```python
from build123d import *

# Parameters (mm, degrees)
CHAMFER1_SIZE          = 1
MOVE_START             = -5
MOVE_FACE1_OUTLINE_R   = 12.65
MOVE_FACE1_OUTLINE_R_2 = 12.5
MOVE_FACE1_OUTLINE_R_3 = 10.5
MOVE_FACE1_OUTLINE_R_4 = 10.35
MOVE_FACE1_DEPTH       = 22
SKETCH2_W              = 3
SKETCH2_H              = 0.5
LPATTERN1_COUNT        = 15
LPATTERN1_PITCH        = 1.25


with BuildPart() as part:
    # Sketch1 → Revolve1 (revolve)
    with BuildSketch(Plane.XY, mode=Mode.PRIVATE) as revolve1_sk:
        with BuildLine():
            Line((0, -15), (0, 17))
            Line((0, 17), (10.5, 17))
            Line((10.5, 17), (10.5, -5))
            Line((10.5, -5), (12.5, -5))
            Line((12.5, -5), (12.5, 9.5))
            Line((12.5, 9.5), (14.696938457, 9.5))
            ThreePointArc((14.696938457, 9.5), (17.047381221, -3.954338567), (9.013878189, -15))
            Line((9.013878189, -15), (0, -15))
        make_face()
    revolve(revolve1_sk.sketch.rotate(Axis((0, -15, 0), (0, 1, 0)), 90), axis=Axis((0, -15, 0), (0, 1, 0)))

    # Chamfer1
    # the kernel refuses this chamfer: 3.367367181, 1 mm, written as the material it takes off along each edge
    with BuildSketch(Plane(origin=(0, 17, 0), x_dir=(0, 0, -1), z_dir=(1, 0, 0))) as chamfer1_piece_1:
        Polygon((10.5 - CHAMFER1_SIZE, 0), (10.5, -CHAMFER1_SIZE), (10.5, 0), align=None)
    revolve(axis=Axis((0, 17, 0), (0, 1, 0)), mode=Mode.SUBTRACT)
    with BuildSketch(Plane(origin=(0, 9.5, 0), x_dir=(0, 0, -1), z_dir=(1, 0, 0))) as chamfer1_piece_2:
        Polygon((12.5, -CHAMFER1_SIZE), (12.5 + CHAMFER1_SIZE, 0), (12.5, 0), align=None)
    revolve(axis=Axis((0, 9.5, 0), (0, 1, 0)), mode=Mode.SUBTRACT)
    with BuildSketch(Plane(origin=(0, 9.5, 0), x_dir=(0, 0, -1), z_dir=(1, 0, 0))) as chamfer1_piece_3:
        with BuildLine():
            Line((14.696938457 - CHAMFER1_SIZE, 0), (15.911300266, -2.214361809))
            ThreePointArc((15.911300266, -2.214361809), (15.375147387, -1.142079038), (14.696938457, 0))
            Line((14.696938457, 0), (14.696938457 - CHAMFER1_SIZE, 0))
        make_face()
    revolve(axis=Axis((0, 9.5, 0), (0, 1, 0)), mode=Mode.SUBTRACT)

    # Move Face1: read off the stored shape, not the designer's step
    # Move Face1 outline → Move Face1 (cut)
    # profile 1 of 2: a face of its own
    with BuildSketch(Plane(origin=(0, 0, 0), x_dir=(1, 0, 0), z_dir=(0, 1, 0)).offset(MOVE_START)):
        Circle(MOVE_FACE1_OUTLINE_R)
        Circle(MOVE_FACE1_OUTLINE_R_2, mode=Mode.SUBTRACT)
    # profile 2 of 2: a face of its own
    with BuildSketch(Plane(origin=(0, 0, 0), x_dir=(1, 0, 0), z_dir=(0, 1, 0)).offset(MOVE_START)):
        Circle(MOVE_FACE1_OUTLINE_R_3)
        Circle(MOVE_FACE1_OUTLINE_R_4, mode=Mode.SUBTRACT)
    extrude(amount=MOVE_FACE1_DEPTH, mode=Mode.SUBTRACT)

    # Sketch2 → Cut-Revolve1 (revolve, cut)
    with BuildSketch(Plane.XY):
        with Locations((11.5, 14.4)):
            Rectangle(SKETCH2_W, SKETCH2_H)
    cut_revolve1 = revolve(axis=Axis((0, 0, 0), (0, 1, 0)), mode=Mode.SUBTRACT)

    # LPattern1: Cut-Revolve1 ×15
    with Locations(*[(0, -i * LPATTERN1_PITCH, 0) for i in range(1, LPATTERN1_COUNT)]):
        add(cut_revolve1, mode=Mode.SUBTRACT)


solid = part.part
```
Check sheet for the modelled part. Datum: model origin and axes. Units: mm. A direction names the side the tool comes from. Give positions to 0.01 mm unless a question says otherwise; leave off trailing zeros. Order: outer loops, then holes, each group sorted by start corner. A loop starts at its lowest first (then second) coordinate and runs counter-clockwise, first axis right, second up. Notation, with made-up numbers: M 2.25,60 L 21.25,60 A14 ccw 21.25,83 Z; hole C -39,43.5 d11. An arc over 180 degrees is marked long. Answer in a Markdown table with one row per item. Add a question column.
Q1. Gauge pin test, flat ends, axial feed: pin 1 Ø1 at (x, z) = (7.5, -10) entering from -Y; pin 2 Ø1.5 at (y, z) = (1.5, -1) entering from -X; pin 3 Ø2 at (x, z) = (13, 7.5) entering from +Y. Record the tip position at first contact, or that the pin passes through.
Q2. Release check for a two-part mould opening along Y. For faces 1 (the cylindrical face through (-2.74, -1.23, 12.35)), 2 (the conical face through (5, 9, -12)), 3 (the cylindrical face through (-2.17, 10.65, 9.76)) record: released by +Y, released by -Y, zero draft, split by the parting line, or undercut.
Q3. Thickness scan on L1, parallel to Z at x = -8.5, y = 2; L2, parallel to X at y = 1.8, z = 0; L3, parallel to X at y = 0, z = -6. Record the ranges inside material, lowest first.
Q4. Access from +Z, -Z, +X, -X, +Y, -Y to the whole of each face (thin tool, end or side, straight path). Record for faces 4 (the cylindrical face through (-2.17, -1.85, 9.76)), 5 (the cylindrical face through (-2.74, 3.77, 12.35)).
Q5. Sectioned sample at A-A, the plane y = -9.5. Record the boundary of the cut face in (x, z), and give its area (3 significant figures).
Verdict:
| question | item | result |
|---|---|---|
| 1 | pin 1 | y = -12.74 |
| 1 | pin 2 | x = -17.47 |
| 1 | pin 3 | y = 9.19 |
| 2 | face 1 | zero draft |
| 2 | face 2 | released by +Y |
| 2 | face 3 | undercut |
| 3 | L1 | -15.17 to -9.84, -5.27 to 5.27, 9.84 to 15.17 |
| 3 | L2 | -17.41 to -13, -10 to 10, 13 to 17.41 |
| 3 | L3 | -16.44 to -11.14, -8.43 to 8.43, 11.14 to 16.44 |
| 4 | face 4 | none |
| 4 | face 5 | +Y |
| 5 | outline | C 0,0 d29.39 |
| 5 | area | 679 mm² |
